Read the model definition and answer for the solid it produces. Units are mm, in the model's axes. A direction names the side the tool comes from. Give positions to 0.01 mm unless a question says otherwise; leave off trailing zeros. Loops run counter-clockwise (first coordinate to the right, second up) from the corner with the lowest first, then second, coordinate; pieces in that order, holes last. Notation, with made-up numbers: (-8.75, -5) - (-0.75, -5) arc R35 ccw to (-0.75, 33) - close; hole circle Ø6 at (-37.75, -37.5). An arc over 180 degrees is marked (long way). Write each question's results on one line, items separated by ' | '. Start each with the question number.
Q1. Determine the mould class of faces 5 (the cylindrical face through (17.34, -7.48, -6.84)), 6 (the flat face through (2.129, 0, -20)), 7 (the flat face through (0, -8, 0)) for opening direction X: +X half, -X half, draft (parallel to the pull), parting line (faces both ways), or undercut.
Q2. For faces 1 (the flat face through (-10, -1.425, -15)), 2 (the flat face through (-11, 0, -20.25)), 3 (the flat face through (-16, -8.495, -6)), 4 (the flat face through (11, 0, -20.25)), determine the directions among +Z, -Z, +X, -X, +Y, -Y from which every point of the face is accessible in a straight line to the end or side of a thin tool.
Q3. Given pin 1 (0.5 mm diameter, centred on y = 0, z = -19.5, fed in from +X); pin 2 (1 mm diameter, centred on x = 0.5, y = -2.5, fed in from +Z); pin 3 (6 mm diameter, centred on x = 6.5, y = -3, fed in from +Z), each flat-ended and moving along its own axis, determine where each tip first touches the part or whether it passes through.
Q4. The part is cut by section B-B, the plane z = -15.5. Write down the section's boundary in (x, y) (3 decimals).
Q5. The part is cut by section A-A, the plane x = 15.75. Write down the section's boundary in (y, z) (3 decimals).
Q6. Find the intervals of material crossed by line 1 (Z direction, x = 15.75, y = -8) (3 decimals); line 2 (X direction, y = -2.25, z = -14); line 3 (Z direction, x = 8, y = -6.25), in increasing order. Write a range as from..to.
Q7. The part is cut by section D-D, the plane x = 9.5. Write down the section's boundary in (y, z) (3 decimals).
Q8. The part is cut by section C-C, the plane y = -4. Write down the section's boundary in (x, z), plus the area to 3 significant figures.
```python
from build123d import *

# Parameters (mm, degrees)
MOTOR_HOLDER_BODY_EXTRUDE_DEPTH          = 13.25
ROLLER_HOLDER_BODY_EXTRUDE_DEPTH         = 7
ALIGNER_4_W                              = 0.4
ALIGNER_4_H                              = 2.5
ALIGNMENT_RAIL_EXTRUDE_DEPTH             = 1
ALIGNER_W                                = 39.5
ALIGNER_H                                = 10.575
ALIGNMENT_WALL_EXTRUDE_DEPTH             = 1
ELECTRODE_GROOVE_CUT_EXTRUDE_DEPTH       = 18.25
FIBRE_GROOVE_CUT_EXTRUDE_DEPTH           = 18.25
ADJUSTMENT_SCREW_HOLES_R                 = 2
ADJUSTMENT_SCREW_HOLES_CUT_EXTRUDE_DEPTH = 2


with BuildPart() as part:
    # MOTOR HOLDER → Motor Holder Body Extrude (new body)
    with BuildSketch(Plane.XY):
        with BuildLine():
            Line((-19.75, -9.5), (19.75, -9.5))
            Line((19.75, -9.5), (19.75, -6.495190528))
            Line((19.75, -6.495190528), (3.75, -6.495190528))
            ThreePointArc((3.75, -6.495190528), (0, -7.5), (-3.75, -6.495190528))
            Line((-3.75, -6.495190528), (-19.75, -6.495190528))
            Line((-19.75, -6.495190528), (-19.75, -9.5))
        make_face()
    extrude(amount=-MOTOR_HOLDER_BODY_EXTRUDE_DEPTH)

    # ROLLER HOLDER → Roller Holder Body Extrude (add)
    with BuildSketch(Plane(origin=(0, 0, -13.25), x_dir=(-1, 0, 0), z_dir=(0, 0, -1))):
        with BuildLine():
            Line((19.75, -9.5), (-19.75, -9.5))
            Line((-19.75, -9.5), (-19.75, -1.425))
            Line((-19.75, -1.425), (-1.5, -1.425))
            Line((-1.5, -1.425), (-1.5, -3))
            ThreePointArc((-1.5, -3), (0, -4.5), (1.5, -3))
            Line((1.5, -3), (1.5, -1.425))
            Line((1.5, -1.425), (19.75, -1.425))
            Line((19.75, -1.425), (19.75, -9.5))
        make_face()
    extrude(amount=ROLLER_HOLDER_BODY_EXTRUDE_DEPTH)

    # ALIGNER<4> → Alignment Rail Extrude (add)
    with BuildSketch(Plane(origin=(0, 0, -20.25), x_dir=(-1, 0, 0), z_dir=(0, 0, -1))):
        with Locations((1.7, -0.175)):
            Rectangle(ALIGNER_4_W, ALIGNER_4_H)
        with Locations((-1.929199775, -0.175)):
            Rectangle(ALIGNER_4_W, ALIGNER_4_H)
    extrude(amount=-ALIGNMENT_RAIL_EXTRUDE_DEPTH)

    # ALIGNER → Alignment Wall Extrude (add)
    with BuildSketch(Plane(origin=(0, 0, -20.25), x_dir=(-1, 0, 0), z_dir=(0, 0, -1))):
        with Locations((0, -4.2125)):
            Rectangle(ALIGNER_W, ALIGNER_H)
    extrude(amount=ALIGNMENT_WALL_EXTRUDE_DEPTH)

    # ELECTRODE GROOVE → Electrode Groove Cut Extrude (cut)
    with BuildSketch(Plane(origin=(19.75, 0, 0), x_dir=(0, 0, -1), z_dir=(1, 0, 0))):
        with BuildLine():
            Line((16.725, -1.425), (16.775, -1.425))
            Line((16.775, -1.425), (16.775, -1.475))
            ThreePointArc((16.775, -1.475), (16.75, -1.5), (16.725, -1.475))
            Line((16.725, -1.475), (16.725, -1.425))
        make_face()
    extrude(amount=-ELECTRODE_GROOVE_CUT_EXTRUDE_DEPTH, mode=Mode.SUBTRACT)

    # FIBRE GROOVE → Fibre Groove Cut Extrude (cut)
    with BuildSketch(Plane.ZY.offset(19.75)):
        with BuildLine():
            Line((-16.85, -1.425), (-16.85, -1.475))
            ThreePointArc((-16.85, -1.475), (-16.75, -1.55698039), (-16.65, -1.475))
            Line((-16.65, -1.475), (-16.65, -1.425))
            Line((-16.65, -1.425), (-16.85, -1.425))
        make_face()
    extrude(amount=-FIBRE_GROOVE_CUT_EXTRUDE_DEPTH, mode=Mode.SUBTRACT)

    # ADJUSTMENT SCREW HOLES → Adjustment Screw Holes Cut Extrude (cut)
    with BuildSketch(Plane(origin=(0, -6.495190528, 0), x_dir=(1, 0, 0), z_dir=(0, 1, 0))):
        with Locations(Location((-15.75, 5.625, 0), (0, 0, 180))):
            Circle(ADJUSTMENT_SCREW_HOLES_R)
        with Locations(Location((15.75, 5.625, 0), (0, 0, 180))):
            Circle(ADJUSTMENT_SCREW_HOLES_R)
    extrude(amount=-ADJUSTMENT_SCREW_HOLES_CUT_EXTRUDE_DEPTH, mode=Mode.SUBTRACT)


solid = part.part
```
Check sheet entries:
1) face 5: undercut | face 6: +X half | face 7: draft
2) face 1: +Z, +X, -X, +Y | face 2: +Z, -X, +Y | face 3: +Y | face 4: +Z, +X, +Y
3) pin 1: stops at x = 2.13 | pin 2: stops at z = -20.25 | pin 3: stops at z = -13.25
4) outline: (-19.75, -9.5) - (19.75, -9.5) - (19.75, -1.425) - (1.5, -1.425) - (1.5, -3) arc R1.5 cw to (-1.5, -3) - (-1.5, -1.425) - (-19.75, -1.425) - close
5) outline: (-9.5, -21.25) - (1.075, -21.25) - (1.075, -20.25) - (-1.425, -20.25) - (-1.425, -16.775) - (-1.475, -16.775) arc R0.025 cw to (-1.475, -16.725) - (-1.425, -16.725) - (-1.425, -13.25) - (-6.495, -13.25) - (-6.495, -7.625) - (-8.495, -7.625) - (-8.495, -3.625) - (-6.495, -3.625) - (-6.495, 0) - (-9.5, 0) - close
6) line 1: z = -21.25..-7.625, -3.625..0 | line 2: x = -19.75..-1.5, 1.5..19.75 | line 3: z = -21.25..-13.25
7) outline: (-9.5, -21.25) - (1.075, -21.25) - (1.075, -20.25) - (-1.425, -20.25) - (-1.425, -16.775) - (-1.475, -16.775) arc R0.025 cw to (-1.475, -16.725) - (-1.425, -16.725) - (-1.425, -13.25) - (-6.495, -13.25) - (-6.495, 0) - (-9.5, 0) - close
8) outline: (-19.75, -21.25) - (19.75, -21.25) - (19.75, -13.25) - (1.12, -13.25) - (1.12, -20.25) - (-1.12, -20.25) - (-1.12, -13.25) - (-19.75, -13.25) - close | area: 300 mm^2
